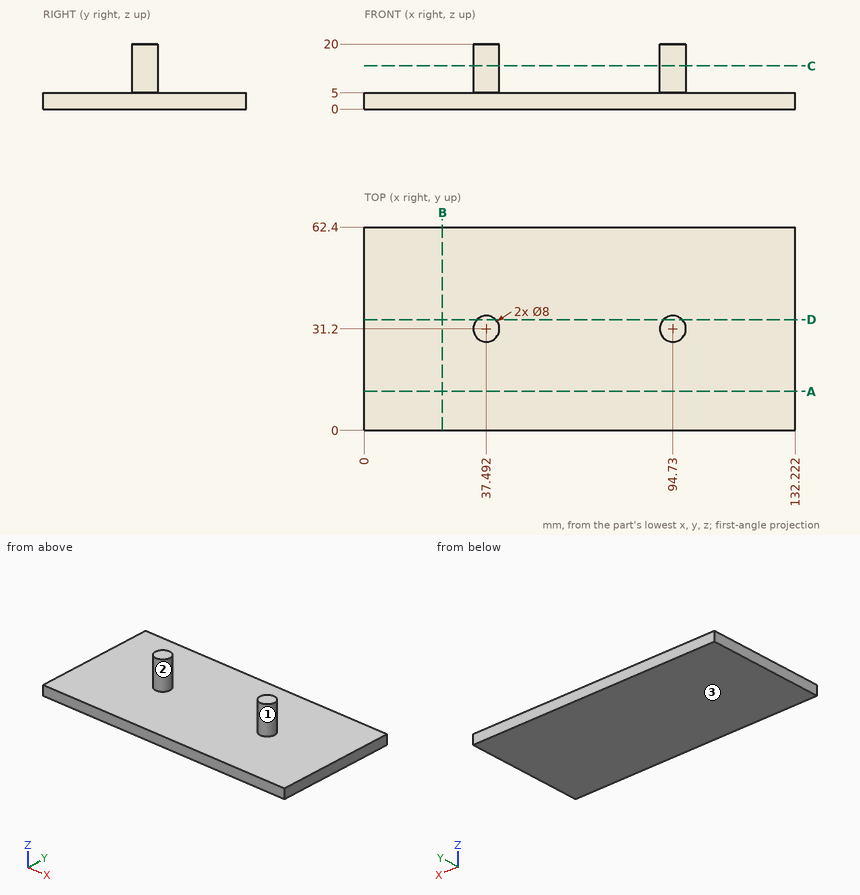
Answer from the drawing. Dimensions are ordinates in mm from the lowest x, y and z of the part. Give positions to 0.01 mm unless a question says otherwise; leave off trailing zeros. Order: outer loops, then holes, each group sorted by start corner. A loop starts at its lowest first (then second) coordinate and runs counter-clockwise, first axis right, second up.
Item 1: Find the intervals of material crossed by probe 1 along Z at (x, y) = (112, 19); probe 2 along X at (y, z) = (33.5, 10.25) (1 decimal); probe 3 along Y at (x, z) = (91.5, 7), in increasing order.
From the geometry:
probe 1: z = 0 to 5
probe 2: x = 34.2 to 40.8, 91.5 to 98
probe 3: y = 28.84 to 33.56
Item 2: For a pull along X with two mould halves and no side action, classify the marked faces 1, 2 and 3 as pulls with the +X half, pulls with the -X half, needs draft (parallel to the pull), parting line crosses it, or undercut.
From the geometry:
face 1: undercut
face 2: undercut
face 3: needs draft
Item 3: The part is cut by section C-C, the plane z = 13.25. Give the vertices of the cut face in (x, y), and give its area (3 significant figures).
From the geometry:
outline: circle Ø8 at (37.49, 31.2); circle Ø8 at (94.73, 31.2)
area: 101 mm2
Item 4: The part is cut by section A-A, the plane y = 12. Give the vertices of the cut face in (x, z).
From the geometry:
outline: (0, 0) - (132.22, 0) - (132.22, 5) - (0, 5) - close
Item 5: The part is cut by section D-D, the plane y = 34. Give the vertices of the cut face in (x, z) (1 decimal).
From the geometry:
outline: (0, 0) - (132.2, 0) - (132.2, 5) - (97.6, 5) - (97.6, 20) - (91.9, 20) - (91.9, 5) - (40.3, 5) - (40.3, 20) - (34.6, 20) - (34.6, 5) - (0, 5) - close
Item 6: The part is cut by section B-B, the plane x = 24. Give the vertices of the cut face in (y, z), and give its area (3 significant figures).
From the geometry:
outline: (0, 0) - (62.4, 0) - (62.4, 5) - (0, 5) - close
area: 312 mm2
Item 7: Given pin 1 Ø3 at (x, y) = (106, 50) entering from +Z; pin 2 Ø3 at (x, z) = (36.5, 11.5) entering from +Y, each flat-ended and moving along its own axis, determine where each tip first touches the part or whether it passes through.
From the geometry:
pin 1: stops at z = 5
pin 2: stops at y = 35.2
